Part print with two shaded views. Sizes in mm from the minimum x, y, z corner. A direction names the side the tool comes from. Give positions to 0.01 mm unless a question says otherwise; leave off trailing zeros. Order: outer loops, then holes, each group sorted by start corner. A loop starts at its lowest first (then second) coordinate and runs counter-clockwise, first axis right, second up. Notation, with made-up numbers: (85, 74) -> (114, 74) arc R30 ccw to (114, 102) -> close; hole circle Ø2 at (-9.5, -6.75). An arc over 180 degrees is marked (long way). Answer as CSV lines item,"result".
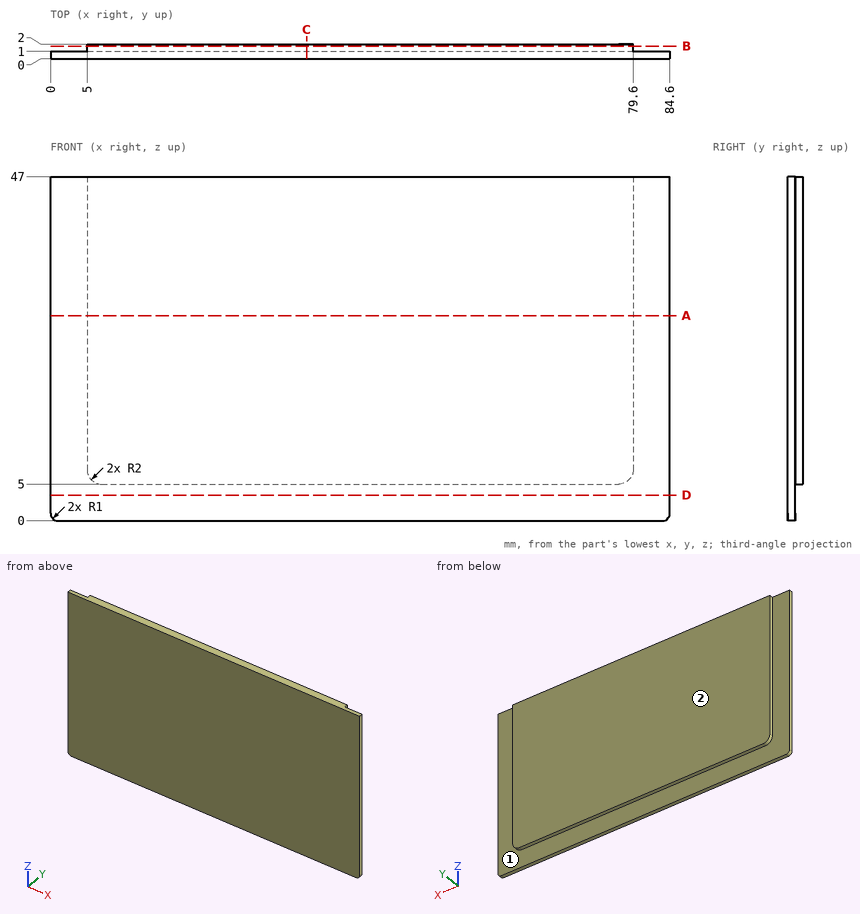
1) Pin check, flat tips, straight feed: P1, Ø0.5, axis at x = 49, y = 1.5, coming from the -Z side; P2, Ø0.8, axis at y = 1.5, z = 25.5, coming from the +X side. Stop position of each tip, or through.
Data:
P1,"stops at z = 5"
P2,"stops at x = 79.6"
2) Band-saw the part on A-A, the plane z = 28. Write the cut outline in (x, y), then the cut area to 3 significant figures.
Data:
outline,"(0, 0) -> (84.6, 0) -> (84.6, 1) -> (79.6, 1) -> (79.6, 2) -> (5, 2) -> (5, 1) -> (0, 1) -> close"
area,"159 mm2"
3) Band-saw the part on D-D, the plane z = 3.5. Write the cut outline in (x, y), then the cut area to 3 significant figures.
Data:
outline,"(0, 0) -> (84.6, 0) -> (84.6, 1) -> (0, 1) -> close"
area,"84.6 mm2"
4) Band-saw the part on C-C, the plane x = 35. Write the cut outline in (y, z).
Data:
outline,"(0, 0) -> (1, 0) -> (1, 5) -> (2, 5) -> (2, 47) -> (0, 47) -> close"
5) Wall check: line 1 along Z through (x, y) = (70, 1.45); line 2 along X through (y, z) = (1.35, 14). Give the ranges that are in metal, low to high. Write a range as [from, to].
Data:
line 1,"z = [5, 47]"
line 2,"x = [5, 79.6]"
6) Band-saw the part on B-B, the plane y = 1.7. Write the cut outline in (x, z).
Data:
outline,"(5, 7) arc R2 ccw to (7, 5) -> (77.6, 5) arc R2 ccw to (79.6, 7) -> (79.6, 47) -> (5, 47) -> close"
7) Which spindle directions (+Z, -Z, +X, -X, +Y, -Y) get a long thin tool onto all of the face, cutting with end or side? Do the marked faces 1 and 2. Say none if no direction does.
Data:
face 1,"-Z, +Y"
face 2,"+Z, -Z, +X, -X, +Y"
